Autodesk Inventor part; units mm, degrees
ref_plane "YZ Plane" through (0, 0, 0) normal (1, 0, 0) x (0, 1, 0)
ref_plane "XZ Plane" through (0, 0, 0) normal (0, 1, 0) x (-1, 0, 0)
ref_plane "XY Plane" through (0, 0, 0) normal (0, 0, 1) x (1, 0, 0)
sketch "Sketch1" plane through (0, 0, 0) normal (0, 1, 0) x (-1, 0, 0)
  circle A0 centre (0, 0) radius 1.4732
  circle A1 centre (0, -28.4988) radius 1.4732
  circle A2 centre (0, 0) radius 5.0165
  circle A3 centre (0, -28.4988) radius 5.0165
  line L0 (5.0165, 0) -> (5.0165, -28.4988)
  line L1 (-5.0165, 0) -> (-5.0165, -28.4988)
  dimension "d0" = 2.9464
  dimension "d2" = 2.9464
  dimension "d3" = 10.033
  dimension "d4" = 10.033
extrude "Extrusion1" add sketch "Sketch1" along normal blind 3.5
sketch "Sketch2" plane through (5.0165, 0, 0) normal (1, 0, 0) x (0, 0, -1)
  line L0 (0, 0) -> (28.4988, 0)
  line L1 (0, 0) -> (5.0292, 0)
  line L2 (28.4988, 0) -> (28.4988, 3.5)
  line L3 (28.4988, 0) -> (23.4696, 0)
  line L4 (23.4696, 0) -> (5.0292, 0)
  line L5 (5.0292, 0) -> (5.0292, -25.7302)
  line L6 (8.2042, -28.9052) -> (20.2946, -28.9052)
  line L7 (23.4696, -25.7302) -> (23.4696, 0)
  line L8 (5.0292, 0) -> (23.4696, 0)
  line L9 (5.0292, 0) -> (11.3792, 0)
  line L10 (23.4696, 0) -> (17.1196, 0)
  line L11 (5.0292, -28.9052) -> (11.3792, -28.9052)
  arc A0 (5.0292, -25.7302) -> (8.2042, -28.9052) centre (8.2042, -25.7302) ccw
  arc A1 (20.2946, -28.9052) -> (23.4696, -25.7302) centre (20.2946, -25.7302) ccw
  line L12 (15.8041, -24.4147) -> (12.694, -24.4147)
  line L13 (12.694, -4.4898) -> (15.8041, -4.4898)
  line L14 (18.9791, -7.6648) -> (18.9791, -21.2397)
  line L15 (9.519, -21.2397) -> (9.519, -7.6648)
  arc A2 (12.694, -4.4898) -> (9.519, -7.6648) centre (12.694, -7.6648) ccw
  arc A3 (9.519, -21.2397) -> (12.694, -24.4147) centre (12.694, -21.2397) ccw
  arc A4 (15.8041, -24.4147) -> (18.9791, -21.2397) centre (15.8041, -21.2397) ccw
  arc A5 (18.9791, -7.6648) -> (15.8041, -4.4898) centre (15.8041, -7.6648) ccw
  point P0 (9.519, -24.4147)
  dimension "d7" = 5.0292
  dimension "d8" = 5.0292
  dimension "d9" = 28.9052
  dimension "d10" = 6.35
  dimension "d14" = 6.35
  dimension "d17" = 3.175
  dimension "d23" = 6.35
  dimension "d25" = 3.175
extrude "Extrusion4" add sketch "Sketch2" along normal blind 3.5
sketch "Sketch4" plane through (5.0165, 0, -5.0292) normal (0, 1, 0) x (1, 0, 0)
  line L0 (0, 0) -> (3.5, 0)
  line L1 (3.5, 15.2654) -> (3.5, 18.4404)
  line L2 (3.5, 0) -> (3.5, 18.4404)
  line L3 (0, 18.4404) -> (3.5, 18.4404)
  line L4 (3.5, 18.4404) -> (0, 18.4404)
  line L5 (0, 18.4404) -> (0, 0)
  line L6 (0, 0) -> (3.5, 0)
  point P0 (-5.0165, -5.0292)
extrude "Extrusion5" add sketch "Sketch4" along normal blind 3.5
fillet "Fillet3" radius 3.175 1 edges at (8.5165, 3.5, -14.2494)
properties part number "frontbackmount"
Work out the finished part from the listing and answer in its coordinate system (mm). A direction names the side the tool comes from. Round coordinates to 2 decimals unless told otherwise and drop trailing zeros. Loops run counter-clockwise (first coordinate to the right, second up) from the corner with the lowest first, then second, coordinate; pieces in that order, holes last. Notation, with made-up numbers: (42, 78.25) -> (71, 78.25) arc R20 ccw to (71, 84.25) -> close; hole circle Ø4 at (13, 78.25). An arc over 180 degrees is marked (long way). Use one line per item in the form item = value.
(1) A tool of negligible diameter and unlimited length cuts with its end or side. For faces 1 (the cylindrical face through (6.742, -23.509, -10.474)), 2 (the flat face through (0, 0, -14)), 3 (the flat face through (5.016, 2, -26)), from which of +Z, -Z, +X, -X, +Y, -Y can it reach the whole face along a straight path? Write none if from no direction.
Answer list:
face_1 = +X, -X
face_2 = +Z, -Z, -X, -Y
face_3 = -Z, +X, +Y, -Y
(2) For a pull along Z with two mould halves and no side action, classify faces 4 (the flat face through (7, -24.415, -14)), 5 (the cylindrical face through (6.742, -27.95, -22.564)), 6 (the cylindrical face through (7.611, 2.545, -14.12)), 7 (the cylindrical face through (6.742, -23.46, -18.074)) as released by +Z, released by -Z, zero draft, split by the parting line, or undercut.
Answer list:
face_4 = undercut
face_5 = released by -Z
face_6 = zero draft
face_7 = undercut
(3) Flat-ended cylindrical pins translate along their axes: P1, Ø2, axis at x = 1.5, z = -28.5, coming from the -Y side; P2, Ø5.5, axis at y = -17, z = -17.5, coming from the -X side; P3, Ø3, axis at y = 1, z = -26, coming from the +X side; P4, Ø8, axis at x = 1, y = -1.5, coming from the +Z side. Find the tip coordinate at first contact, or state that the pin passes through.
Answer list:
P1 = 0
P2 = 5.02
P3 = 5.02
P4 = 5.02
(4) Find section A-A on x = 0. Give the vertices of the cut face in (y, z).
Answer list:
outline = (0, -33.52) -> (3.5, -33.52) -> (3.5, -29.97) -> (0, -29.97) -> close; (0, -27.03) -> (3.5, -27.03) -> (3.5, -1.47) -> (0, -1.47) -> close; (0, 1.47) -> (3.5, 1.47) -> (3.5, 5.02) -> (0, 5.02) -> close
(5) Find section C-C on x = 7.75. Give the vertices of the cut face in (y, z) (3 decimals), then the cut area to 3 significant figures.
Answer list:
outline = (-28.905, -20.295) arc R3.175 ccw to (-25.73, -23.47) -> (2.394, -23.47) -> (2.394, -5.029) -> (-25.73, -5.029) arc R3.175 ccw to (-28.905, -8.204) -> close; hole (-24.415, -15.804) arc R3.175 ccw to (-21.24, -18.979) -> (-7.665, -18.979) arc R3.175 ccw to (-4.49, -15.804) -> (-4.49, -12.694) arc R3.175 ccw to (-7.665, -9.519) -> (-21.24, -9.519) arc R3.175 ccw to (-24.415, -12.694) -> close
area = 393 mm2
(6) Find section B-B on y = -19. Give the vertices of the cut face in (x, z).
Answer list:
outline = (5.02, -23.47) -> (8.52, -23.47) -> (8.52, -18.98) -> (5.02, -18.98) -> close; (5.02, -9.52) -> (8.52, -9.52) -> (8.52, -5.03) -> (5.02, -5.03) -> close
(7) Straight lines are drawn through the part: line 1 (Z direction, x = 0, y = 2.25); line 2 (Y direction, x = -3.5, z = -6.5); line 3 (X direction, y = -2, z = -19.5). For each, find the intervals that lie inside material, in ascending order.
Answer list:
line_1 = -33.52 to -29.97, -27.03 to -1.47, 1.47 to 5.02
line_2 = 0 to 3.5
line_3 = 5.02 to 8.52
